from build123d import *

# Parameters (mm, degrees)
SKETCH1_W          = 5.842
SKETCH1_H          = 3.175
SKETCH1_W_2        = 3.175
SKETCH1_H_2        = 31.75
SKETCH2_W          = 4.7625
SKETCH2_H          = 25.4
CUT_EXTRUDE1_DEPTH = 25.4
SKETCH3_W          = 17.78
SKETCH3_H          = 3.175
CUT_EXTRUDE2_DEPTH = 25.4


with BuildPart() as part:
    # Sketch1 → Revolve1 (revolve)
    with BuildSketch(Plane.XY, mode=Mode.PRIVATE) as revolve1_sk:
        with Locations((6.096, 14.2875)):
            Rectangle(SKETCH1_W, SKETCH1_H)
        with Locations((10.6045, 0)):
            Rectangle(SKETCH1_W_2, SKETCH1_H_2)
    revolve(revolve1_sk.sketch.rotate(Axis((0, 0, 0), (0, 1, 0)), 90), axis=Axis((0, 0, 0), (0, 1, 0)))

    # Sketch2 → Cut-Extrude1 (cut, symmetric)
    with BuildSketch(Plane.XY):
        Rectangle(SKETCH2_W, SKETCH2_H)
    extrude(amount=CUT_EXTRUDE1_DEPTH, both=True, mode=Mode.SUBTRACT)

    # Sketch3 → Cut-Extrude2 (cut, symmetric)
    with BuildSketch(Plane(origin=(0, 0, 0), x_dir=(0, 0, -1), z_dir=(1, 0, 0))):
        with Locations((0, -12.7)):
            Rectangle(SKETCH3_W, SKETCH3_H)
        with Locations((0, -7.9375)):
            Rectangle(SKETCH3_W, SKETCH3_H)
        with Locations((0, -3.175)):
            Rectangle(SKETCH3_W, SKETCH3_H)
        with Locations((0, 1.5875)):
            Rectangle(SKETCH3_W, SKETCH3_H)
        with Locations((0, 6.35)):
            Rectangle(SKETCH3_W, SKETCH3_H)
    extrude(amount=CUT_EXTRUDE2_DEPTH, both=True, mode=Mode.SUBTRACT)


solid = part.part
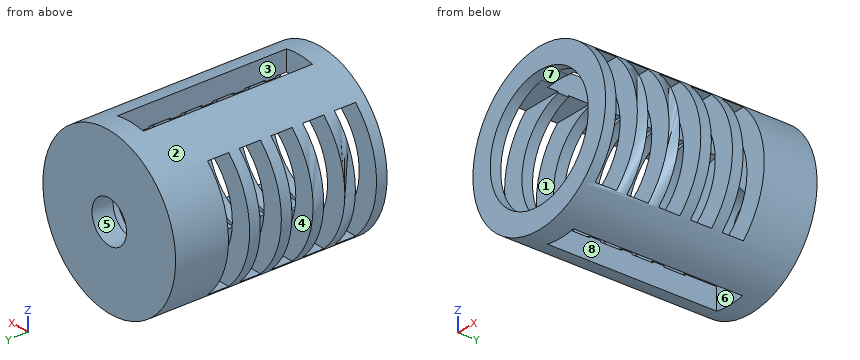
Geometry check sheet. Reference: the model listing, model coordinates, mm. Face numbers are marked on the shaded views. A direction names the side the tool comes from. Give positions to 0.01 mm unless a question says otherwise; leave off trailing zeros. Order: outer loops, then holes, each group sorted by start corner. A loop starts at its lowest first (then second) coordinate and runs counter-clockwise, first axis right, second up. Notation, with made-up numbers: M 2,-9.75 L 14,-9.75 A25 cw 14,16.25 Z; hole C 3.25,-28 d2. An arc over 180 degrees is marked long. Use a Markdown table: item, result.
Item 1: Tool access check on the marked faces 4, 5, 6, 7 and 8. Record the directions out of +Z, -Z, +X, -X, +Y, -Y that give a thin tool (end or side, any length) a straight path to the whole face; none if there is none.
Answers follow:
| item | result |
|---|---|
| face 4 | +X, -X |
| face 5 | +Y, -Y |
| face 6 | none |
| face 7 | -Y |
| face 8 | +Z, -Z |
Item 2: Depth check by flat-ended pin: P1, Ø3, axis at x = 0, z = 2.5, coming from the -Y side; P2, Ø5, axis at y = 10, z = 3.5, coming from the -X side; P3, Ø10, axis at y = -6, z = 8, coming from the +X side. Enter the tip coordinate at first touch or a pass-through.
Answers follow:
| item | result |
|---|---|
| P1 | stops at y = 12.7 |
| P2 | stops at x = -12.15 |
| P3 | stops at x = 11.82 |
Item 3: Draft check along Z on the marked faces 1, 2 and 3. Enter one of: +Z half, -Z half, draft (parallel to the pull), parting line (faces both ways), or undercut.
Answers follow:
| item | result |
|---|---|
| face 1 | undercut |
| face 2 | parting line |
| face 3 | draft |
Item 4: Material ranges on line 1 along X through (y, z) = (13.5, 0) (3 decimals); line 2 along Y through (x, z) = (-4.5, -0.75) (3 decimals); line 3 along X through (y, z) = (11, -10.5), recorded low to high.
Answers follow:
| item | result |
|---|---|
| line 1 | x = -12.192 to -3.175, 3.175 to 12.192 |
| line 2 | y = 12.7 to 15.875 |
| line 3 | x = -6.2 to -2.38, 2.38 to 6.2 |
Item 5: Section check B-B (y = 1). Record the cut outline in (x, z).
Answers follow:
| item | result |
|---|---|
| outline | M -8.34,-8.89 A12.19 ccw -2.38,-11.96 L -2.38,-8.89 Z; M -8.34,8.89 L -2.38,8.89 L -2.38,11.96 A12.19 ccw Z; M 2.38,-11.96 A12.19 ccw 8.34,-8.89 L 2.38,-8.89 Z; M 2.38,8.89 L 8.34,8.89 A12.19 ccw 2.38,11.96 Z |
Item 6: Section check C-C (y = 12). Record the cut outline in (x, z).
Answers follow:
| item | result |
|---|---|
| outline | M -2.38,-11.96 L -2.38,-8.7 A9.02 cw -2.38,8.7 L -2.38,11.96 A12.19 ccw Z; M 2.38,-11.96 A12.19 ccw 2.38,11.96 L 2.38,8.7 A9.02 cw 2.38,-8.7 Z |
Item 7: Section check D-D (z = 0). State how many separate pieces and enclosed holes the cut face has, and give its area (3 significant figures).
Answers follow:
| item | result |
|---|---|
| separate pieces | 12 |
| enclosed holes | 0 |
| area | 138 mm2 |
Item 8: Section check A-A (x = 0). Record the cut outline in (y, z) (3 decimals), and give its area (3 significant figures).
Answers follow:
| item | result |
|---|---|
| outline | M -15.875,-12.192 L -12.7,-12.192 L -12.7,-9.017 L -15.875,-9.017 Z; M -15.875,9.017 L -12.7,9.017 L -12.7,12.192 L -15.875,12.192 Z; M 12.7,-12.192 L 15.875,-12.192 L 15.875,-3.175 L 12.7,-3.175 Z; M 12.7,3.175 L 15.875,3.175 L 15.875,12.192 L 12.7,12.192 Z |
| area | 77.4 mm2 |
